For this review, take the finished solid that the model builds, in its own axes (mm). Coordinates: 2 decimals unless noted, no trailing zeros. Order: outer loops, then holes, each group sorted by start corner. A loop starts at its lowest first (then second) coordinate and runs counter-clockwise, first axis right, second up. Notation, with made-up numbers: M -39,34 L -30,34 A26 cw -30,48 Z; hole C -37,-36.5 d3. An arc over 180 degrees is marked long. Use one line per item in the form item = value. Start each with the question number.
Autodesk Inventor part; units mm, degrees
ref_plane "YZ Plane" through (0, 0, 0) normal (1, 0, 0) x (0, 1, 0)
ref_plane "XZ Plane" through (0, 0, 0) normal (0, 1, 0) x (-1, 0, 0)
ref_plane "XY Plane" through (0, 0, 0) normal (0, 0, 1) x (1, 0, 0)
sketch "スケッチ1" plane through (0, 0, 0) normal (0, 0, 1) x (1, 0, 0)
  line L0 (-72.5, -28) -> (72.5, -28)
  line L1 (72.5, -28) -> (72.5, 28)
  line L2 (72.5, 28) -> (-72.5, 28)
  line L3 (-72.5, 28) -> (-72.5, -28)
  point P0 (0, 0)
  point P1 (0, -28)
  point P2 (-72.5, 0)
  dimension "d0" = 145
  dimension "d1" = 56
extrude "押し出し1" add sketch "スケッチ1" along normal blind 15
sketch "スケッチ3" plane through (0, 0, 15) normal (0, 0, 1) x (1, 0, 0)
  point P0 (0, 0)
  point P1 (-21, 0)
  point P2 (21, 0)
  dimension "d9" = 21
  dimension "d10" = 21
hole "穴1" at (-21, 0, 15) at (21, 0, 15) direction (0, 0, -1) diameter 4.134 end through all
sketch "スケッチ4" plane through (0, 0, 0) normal (0, 0, -1) x (-1, 0, 0)
  line L0 (-72.5, -28) -> (-72.5, 28)
  point P0 (0, 0)
  point P1 (-51.5, 0)
  point P2 (-72.5, 0)
  dimension "d18" = 21
hole "穴2" at (51.5, 0, 0) direction (0, 0, 1) diameter 4.134 end through all
pattern_linear "矩形状パターン1" count 3 spacing 52 along (-1, 0, 0) of "穴2"
sketch "スケッチ5" plane through (0, 0, 0) normal (0, 0, -1) x (-1, 0, 0)
  circle A0 centre (52.5, 0) radius 2.067
  circle A1 centre (0.5, 0) radius 2.067
  point P0 (0, 0)
  point P1 (52.5, -24)
  point P2 (0.5, -24)
  dimension "d29" = 24
hole "穴3" at (-52.5, -24, 0) at (-0.5, -24, 0) direction (0, 0, 1) diameter 5 end through all
chamfer "面取り1" distance 1 angle 45 4 edges at (-72.5, -28, 7.5) (-72.5, 28, 7.5) (72.5, -28, 7.5) (72.5, 28, 7.5)
properties part number "02" material "A5052"
1. Consider section B-B, the plane x = 51.5. Write out the cut boundary in (y, z), plus the area to 3 significant figures.
2. To check wall thickness, follow line 1 (X direction, y = 0, z = 9.5); line 2 (X direction, y = -24, z = 10.5); line 3 (Y direction, x = -52.5, z = 12). State the ranges of each line that lie inside material, in increasing order.
3. Consider section D-D, the plane x = -52.5. Write out the cut boundary in (y, z), plus the area to 3 significant figures.
4. The part is to be moulded in two halves that separate along X. For faces 1 (the cylindrical face through (-54.55, -0.27, 7.6)), 2 (the flat face through (-1, -28, 7)), 3 (the cylindrical face through (49.45, -0.27, 7.6)), 4 (the flat face through (72.5, 0, 7)), say which applies: pulls with the +X half, pulls with the -X half, needs draft (parallel to the pull), parting line crosses it, or undercut.
5. Consider section C-C, the plane y = 0. Write out the cut boundary in (x, z).
6. Consider section A-A, the plane y = -24. Write out the cut boundary in (x, z), plus the area to 4 significant figures.
Answers follow:
q1.outline = M -28,0 L -2.07,0 L -2.07,15 L -28,15 Z; M 2.07,0 L 28,0 L 28,15 L 2.07,15 Z
q1.area = 778 mm²
q2.line_1 = -72.5 to -54.57, -50.43 to -23.07, -18.93 to -2.57, 1.57 to 18.93, 23.07 to 49.43, 53.57 to 72.5
q2.line_2 = -72.5 to -55, -50 to -3, 2 to 72.5
q2.line_3 = -28 to -26.5, -21.5 to -2.07, 2.07 to 28
q3.outline = M -28,0 L -26.5,0 L -26.5,15 L -28,15 Z; M -21.5,0 L -2.07,0 L -2.07,15 L -21.5,15 Z; M 2.07,0 L 28,0 L 28,15 L 2.07,15 Z
q3.area = 703 mm²
q4.face_1 = undercut
q4.face_2 = needs draft
q4.face_3 = undercut
q4.face_4 = pulls with the +X half
q5.outline = M -72.5,0 L -54.57,0 L -54.57,15 L -72.5,15 Z; M -50.43,0 L -23.07,0 L -23.07,15 L -50.43,15 Z; M -18.93,0 L -2.57,0 L -2.57,15 L -18.93,15 Z; M 1.57,0 L 18.93,0 L 18.93,15 L 1.57,15 Z; M 23.07,0 L 49.43,0 L 49.43,15 L 23.07,15 Z; M 53.57,0 L 72.5,0 L 72.5,15 L 53.57,15 Z
q6.outline = M -72.5,0 L -55,0 L -55,15 L -72.5,15 Z; M -50,0 L -3,0 L -3,15 L -50,15 Z; M 2,0 L 72.5,0 L 72.5,15 L 2,15 Z
q6.area = 2,025 mm²
